Drawing for the job (mm, zero at the part's lowest x, y, z). A direction names the side the tool comes from. Round coordinates to 2 decimals unless told otherwise and drop trailing zeros. Order: outer loops, then holes, each group sorted by start corner. A loop starts at its lowest first (then second) coordinate and runs counter-clockwise, first axis right, second up. Notation, with made-up numbers: (-20.5, -15.5) -> (9.5, -15.5) arc R22 cw to (9.5, 17.5) -> close; hole circle Ø3 at (2.5, 13.25). An arc over 180 degrees is marked (long way). Use CSV: the item, a comma, the result in double quotes.
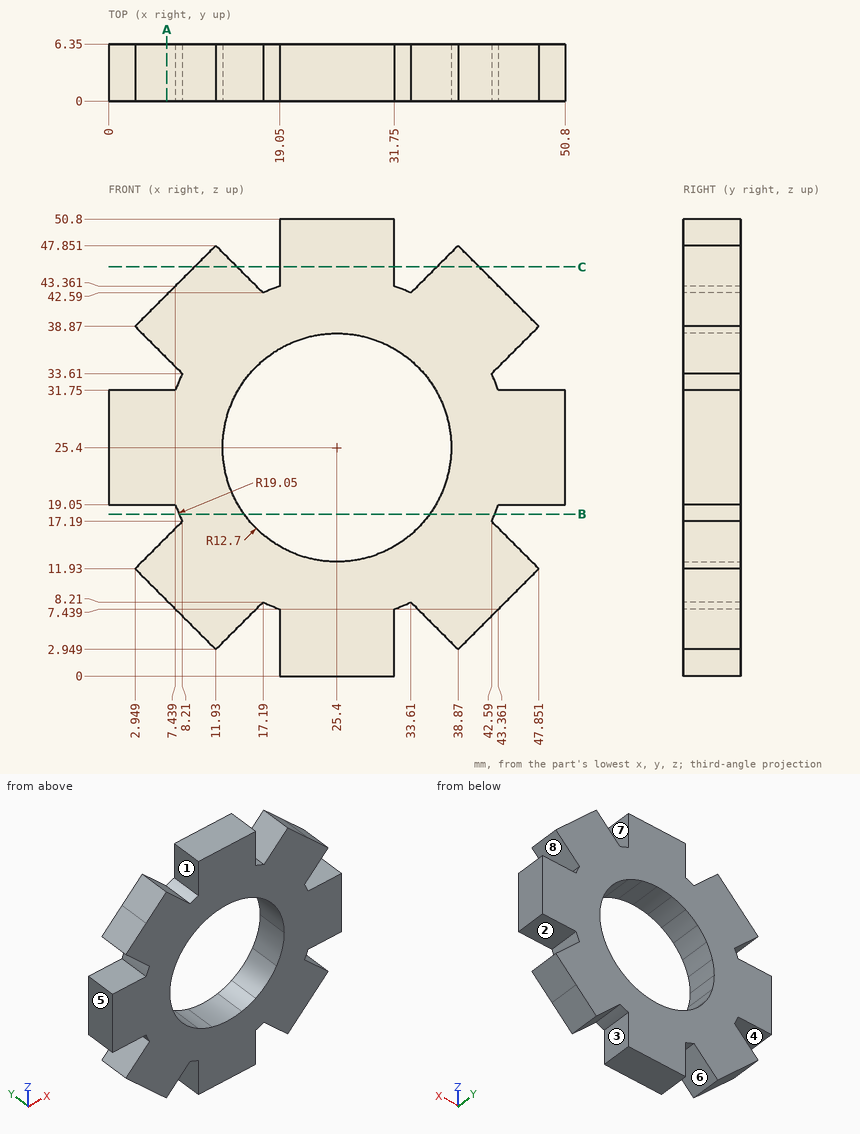
Q1. Cut at A-A (x = 6.5). Give the cut face in (y, z).
From the geometry:
outline,"(0, 8.38) -> (6.35, 8.38) -> (6.35, 15.48) -> (0, 15.48) -> close; (0, 19.05) -> (6.35, 19.05) -> (6.35, 31.75) -> (0, 31.75) -> close; (0, 35.32) -> (6.35, 35.32) -> (6.35, 42.42) -> (0, 42.42) -> close"
Q2. Pin check, flat tips, straight feed: pin 1 (1.9 mm diameter, centred on y = 3.5, z = 2.5, fed in from +X); pin 2 (1.9 mm diameter, centred on x = 5.5, y = 2, fed in from -Z); pin 3 (1.5 mm diameter, centred on y = 4.5, z = 34, fed in from -X). Stop position of each tip, or through.
From the geometry:
pin 1,"stops at x = 39.37"
pin 2,"stops at z = 8.43"
pin 3,"stops at x = 7.07"
Q3. Mould opens along X. For the marked faces 5, 6, 7 and 8 say: +X half, -X half, draft (parallel to the pull), parting line (faces both ways), or undercut.
From the geometry:
face 5,"-X half"
face 6,"undercut"
face 7,"undercut"
face 8,"+X half"
Q4. Probe line 1 along Z through (x, y) = (46, 3.5); line 2 along Z through (x, y) = (47.5, 4.5); line 3 along X through (y, z) = (4.75, 44.5). List the from-to ranges inside material, lowest first.
From the geometry:
line 1,"z = 10.08 to 13.78, 19.05 to 31.75, 37.02 to 40.72"
line 2,"z = 11.58 to 12.28, 19.05 to 31.75, 38.52 to 39.22"
line 3,"x = 8.58 to 15.28, 19.05 to 31.75, 35.52 to 42.22"
Q5. Cut at B-B (z = 18). Give the cut face in (x, y).
From the geometry:
outline,"(7.85, 0) -> (15.08, 0) -> (15.08, 6.35) -> (7.85, 6.35) -> close; (35.72, 0) -> (42.95, 0) -> (42.95, 6.35) -> (35.72, 6.35) -> close"
Q6. Which spindle directions (+Z, -Z, +X, -X, +Y, -Y) get a long thin tool onto all of the face, cutting with end or side? Do the marked faces 1, 2, 3 and 4. Say none if no direction does.
From the geometry:
face 1,"+Z, +Y, -Y"
face 2,"+X, +Y, -Y"
face 3,"-Z, +Y, -Y"
face 4,"-X, +Y, -Y"
Q7. Cut at C-C (z = 45.5). Give the cut face in (x, y), plus the area to 3 significant figures.
From the geometry:
outline,"(9.58, 0) -> (14.28, 0) -> (14.28, 6.35) -> (9.58, 6.35) -> close; (19.05, 0) -> (31.75, 0) -> (31.75, 6.35) -> (19.05, 6.35) -> close; (36.52, 0) -> (41.22, 0) -> (41.22, 6.35) -> (36.52, 6.35) -> close"
area,"140 mm²"
